Check sheet for the modelled part. Datum: model origin and axes. Units: mm. A direction names the side the tool comes from. Give positions to 0.01 mm unless a question says otherwise; leave off trailing zeros. Order: outer loops, then holes, each group sorted by start corner. A loop starts at its lowest first (then second) coordinate and runs counter-clockwise, first axis right, second up.
```python
from build123d import *

# Parameters (mm, degrees)
SKETCH1_W           = 40
SKETCH1_H           = 42
BOSS_EXTRUDE1_DEPTH = 0.6
SKETCH3_R           = 7.5
CUT_EXTRUDE1_DEPTH  = 59.012412465
SKETCH4_W           = 40
SKETCH4_H           = 1.2
BOSS_EXTRUDE2_DEPTH = 22
SKETCH5_R           = 1.5
CUT_EXTRUDE2_DEPTH  = 62.444283705
FILLET1_R           = 1


with BuildPart() as part:
    # Sketch1 → Boss-Extrude1 (new, symmetric)
    with BuildSketch(Plane(origin=(0, 0, 0), x_dir=(1, 0, 0), z_dir=(0, 1, 0))):
        with Locations((20, 21)):
            Rectangle(SKETCH1_W, SKETCH1_H)
    extrude(amount=BOSS_EXTRUDE1_DEPTH, both=True)

    # Sketch3 → Cut-Extrude1 (cut, through all)
    with BuildSketch(Plane(origin=(0, 0.6, 0), x_dir=(1, 0, 0), z_dir=(0, 1, 0))):
        with Locations(Location((20, 21, 0), (0, 0, 270))):
            Circle(SKETCH3_R)
    extrude(amount=-CUT_EXTRUDE1_DEPTH, mode=Mode.SUBTRACT)

    # Sketch4 → Boss-Extrude2 (add)
    with BuildSketch(Plane(origin=(0, 0.6, 0), x_dir=(1, 0, 0), z_dir=(0, 1, 0))):
        with Locations((20, 0.6)):
            Rectangle(SKETCH4_W, SKETCH4_H)
    extrude(amount=BOSS_EXTRUDE2_DEPTH)

    # Sketch5 → Cut-Extrude2 (cut, through all)
    with BuildSketch(Plane(origin=(0, 0, -1.2), x_dir=(-1, 0, 0), z_dir=(0, 0, -1))):
        with Locations((-36, 17.6)):
            Circle(SKETCH5_R)
        with Locations((-36, 5.6)):
            Circle(SKETCH5_R)
        with Locations((-4, 17.6)):
            Circle(SKETCH5_R)
        with Locations((-4, 5.6)):
            Circle(SKETCH5_R)
    extrude(amount=-CUT_EXTRUDE2_DEPTH, mode=Mode.SUBTRACT)

    # Fillet1
    fillet1_edges = [part.edges().sort_by_distance(p)[0] for p in [
        (20, 0.6, -1.2),
    ]]
    fillet(fillet1_edges, radius=FILLET1_R)


solid = part.part
```
(1) Thickness scan on L1, parallel to Y at x = 4, z = -0.35; L2, parallel to Z at x = 5, y = 2.75; L3, parallel to Y at x = 22, z = -33.5. Record the ranges inside material, lowest first.
(2) Tool access check on faces 5 (the face through (37.11, 18.61, -0.61)), 6 (the face through (20, 0.6, -31)). Record the directions out of +Z, -Z, +X, -X, +Y, -Y that give a thin tool (end or side, any length) a straight path to the whole face; none if there is none.
(3) Release check for a two-part mould opening along Z. For faces 1 (the face through (40, 0, -12)), 2 (the face through (20, 11, 0)), 3 (the face through (20, 0, -42)), 4 (the face through (25.1, 0, -26.5)) record: released by +Z, released by -Z, zero draft, split by the parting line, or undercut.
(4) Sectioned sample at A-A (x = 36). Enter the section's corners in (y, z).
(5) Sectioned sample at C-C (x = 20). Enter the section's corners in (y, z), plus the area to 3 significant figures.
(6) Sectioned sample at D-D (z = -17). Enter the section's corners in (x, y).
(7) Go/stop test with flat-tipped pins: P1, Ø1.8, axis at x = 36, y = 5.6, coming from the -Z side; P2, Ø5, axis at x = 36, y = 17.6, coming from the -Z side; P3, Ø20, axis at x = 24, z = -27.5, coming from the +Y side. Record where each tip stops, or that it passes through.
(8) Sectioned sample at B-B (y = 17.6). Enter the section's corners in (x, z).
Values follow:
1. L1: y = -0.6 to 4.1, 7.1 to 16.1, 19.1 to 22.6
1. L2: z = -1.2 to 0
1. L3: y = -0.6 to 0.6
2. face 5: +Z, -Z
2. face 6: -Z, +X, -X, +Y
3. face 1: zero draft
3. face 2: released by +Z
3. face 3: released by -Z
3. face 4: undercut
4. outline: (-0.6, -42) - (0.6, -42) - (0.6, -2.2) arc R1 cw to (1.6, -1.2) - (4.1, -1.2) - (4.1, 0) - (-0.6, 0) - close; (7.1, -1.2) - (16.1, -1.2) - (16.1, 0) - (7.1, 0) - close; (19.1, -1.2) - (22.6, -1.2) - (22.6, 0) - (19.1, 0) - close
5. outline: (-0.6, -42) - (0.6, -42) - (0.6, -28.5) - (-0.6, -28.5) - close; (-0.6, -13.5) - (0.6, -13.5) - (0.6, -2.2) arc R1 cw to (1.6, -1.2) - (22.6, -1.2) - (22.6, 0) - (-0.6, 0) - close
5. area: 59.0 mm2
6. outline: (0, -0.6) - (13.66, -0.6) - (13.66, 0.6) - (0, 0.6) - close; (26.34, -0.6) - (40, -0.6) - (40, 0.6) - (26.34, 0.6) - close
7. P1: passes through
7. P2: stops at z = -1.2
7. P3: stops at y = 0.6
8. outline: (0, -1.2) - (2.5, -1.2) - (2.5, 0) - (0, 0) - close; (5.5, -1.2) - (34.5, -1.2) - (34.5, 0) - (5.5, 0) - close; (37.5, -1.2) - (40, -1.2) - (40, 0) - (37.5, 0) - close
